```python
from build123d import *

# Parameters (mm, degrees)
SKETCH2_R          = 2
CUT_EXTRUDE1_DEPTH = 34.824916851
CIRPATTERN1_COUNT  = 2
CIRPATTERN1_ANGLE  = 90


with BuildPart() as part:
    # Sketch1 → Revolve1 (revolve)
    with BuildSketch(Plane.XY, mode=Mode.PRIVATE) as revolve1_sk:
        Polygon((-4, 0), (-4, 18), (-20.25, 18), (-20.25, 16), (-17, 16), (-17, 9), (-20.25, 9), (-20.25, 7), (-10, 7), (-10, 0), align=None)
    revolve(revolve1_sk.sketch.rotate(Axis((0, 0, 0), (0, 1, 0)), 270), axis=Axis((0, 0, 0), (0, 1, 0)))

    # Sketch2 → Cut-Extrude1 (cut, through all)
    with BuildSketch(Plane.XY):
        with Locations(Location((0, 3.5, 0), (0, 0, 90))):
            Circle(SKETCH2_R)
    cut_extrude1 = extrude(amount=-CUT_EXTRUDE1_DEPTH, mode=Mode.SUBTRACT)

    # CirPattern1: Cut-Extrude1 ×2 about axis
    cirpattern1_axis = Axis((0, 0, 0), (0, 1, 0))
    for i in range(1, CIRPATTERN1_COUNT):
        add(cut_extrude1.rotate(cirpattern1_axis, i * CIRPATTERN1_ANGLE / (CIRPATTERN1_COUNT - 1)), mode=Mode.SUBTRACT)


solid = part.part
```
The model under review builds one solid part; all positions refer to its coordinate system, in mm. A direction names the side the tool comes from. Round coordinates to 2 decimals unless told otherwise and drop trailing zeros. Loops run counter-clockwise (first coordinate to the right, second up) from the corner with the lowest first, then second, coordinate; pieces in that order, holes last. Notation, with made-up numbers: (58.25, -20) - (90.25, -20) arc R9 ccw to (90.25, -9) - close; hole circle Ø11 at (1.25, -6). An arc over 180 degrees is marked (long way). Use a Markdown table: item, result. Add a question column.
Q1. Add section D-D (z = 14.5). State the section outline as (x, y) points, plus the area to 3 significant figures.
Q2. The part is to be moulded in two halves that separate along Y. For faces 6 (the face through (4.2, 18, -0.3)), 7 (the face through (-17, 8, -11)), 8 (the face through (-17, 16, 5)), 9 (the face through (-0.1, 0, -4.3)), say which applies: pulls with the +Y half, pulls with the -Y half, needs draft (parallel to the pull), parting line crosses it, or undercut.
Q3. Add section B-B (x = 3). State the section outline as (y, z) points, plus the area to 3 significant figures.
Q4. Insertion check: pin 1 Ø4.5 at (y, z) = (3.5, 0) entering from +X; pin 2 Ø1.5 at (x, z) = (-11, -7.5) entering from -Y; pin 3 Ø5 at (x, y) = (0, 3.5) entering from -Z; pin 4 Ø1.5 at (y, z) = (2.5, 11.5) entering from +X. Each pin has a flat end and moves straight along its axis. Give the tip position at first contact, or say it passes through.
Q5. Add section A-A (z = 0). State the section outline as (x, y) points.
Q6. Machinability: for faces 1 (the face through (-6.689, 3.24, 1.983)), 2 (the face through (-17, 17, -11)), 3 (the face through (-1.983, 3.24, -6.686)), 4 (the face through (9.76, 3.45, 2.17)), 5 (the face through (-17, 9, -5)), which of the approach directions +Z, -Z, +X, -X, +Y, -Y give a long, thin tool a straight path to every point of the face, cutting with its end or side? Answer none if there is none.
Q7. For probe 1 along X at (y, z) = (4.25, 0); probe 2 along X at (y, z) = (11.25, 0.5); probe 3 along Y at (x, z) = (7, 12), list the stretches that pass through material, from the lowest coordinate up.
Q8. Add section C-C (y = 3.5). State the section outline as (x, z) points.
Worked answers:
| question | item | result |
|---|---|---|
| 1 | outline | (-14.14, 7) - (14.14, 7) - (14.14, 9) - (8.87, 9) - (8.87, 16) - (14.14, 16) - (14.14, 18) - (-14.14, 18) - (-14.14, 16) - (-8.87, 16) - (-8.87, 9) - (-14.14, 9) - close |
| 1 | area | 237 mm² |
| 2 | face 6 | pulls with the +Y half |
| 2 | face 7 | needs draft |
| 2 | face 8 | undercut |
| 2 | face 9 | pulls with the -Y half |
| 3 | outline | (0, -9.54) - (7, -9.54) - (7, -20.03) - (9, -20.03) - (9, -16.73) - (16, -16.73) - (16, -20.03) - (18, -20.03) - (18, -2.65) - (0, -2.65) - close; (0, 2.65) - (18, 2.65) - (18, 20.03) - (16, 20.03) - (16, 16.73) - (9, 16.73) - (9, 20.03) - (7, 20.03) - (7, 9.54) - (0, 9.54) - close |
| 3 | area | 433 mm² |
| 4 | pin 1 | x = 10 |
| 4 | pin 2 | y = 7 |
| 4 | pin 3 | z = -10 |
| 4 | pin 4 | through |
| 5 | outline | (-20.25, 7) - (-10, 7) - (-10, 5.5) - (-4, 5.5) - (-4, 18) - (-20.25, 18) - (-20.25, 16) - (-17, 16) - (-17, 9) - (-20.25, 9) - close; (-10, 0) - (-4, 0) - (-4, 1.5) - (-10, 1.5) - close; (4, 0) - (10, 0) - (10, 7) - (20.25, 7) - (20.25, 9) - (17, 9) - (17, 16) - (20.25, 16) - (20.25, 18) - (4, 18) - close |
| 6 | face 1 | -X |
| 6 | face 2 | +Y, -Y |
| 6 | face 3 | -Z |
| 6 | face 4 | -Y |
| 6 | face 5 | none |
| 7 | probe 1 | 4 to 10 |
| 7 | probe 2 | -16.99 to -3.97, 3.97 to 16.99 |
| 7 | probe 3 | 7 to 18 |
| 8 | outline | (-9.8, -2) arc R10 ccw to (-2, -9.8) - (-2, -3.46) arc R4 cw to (-3.46, -2) - close; (-9.8, 2) - (-3.46, 2) arc R4 cw (long way) to (2, -3.46) - (2, -9.8) arc R10 ccw (long way) to start |
